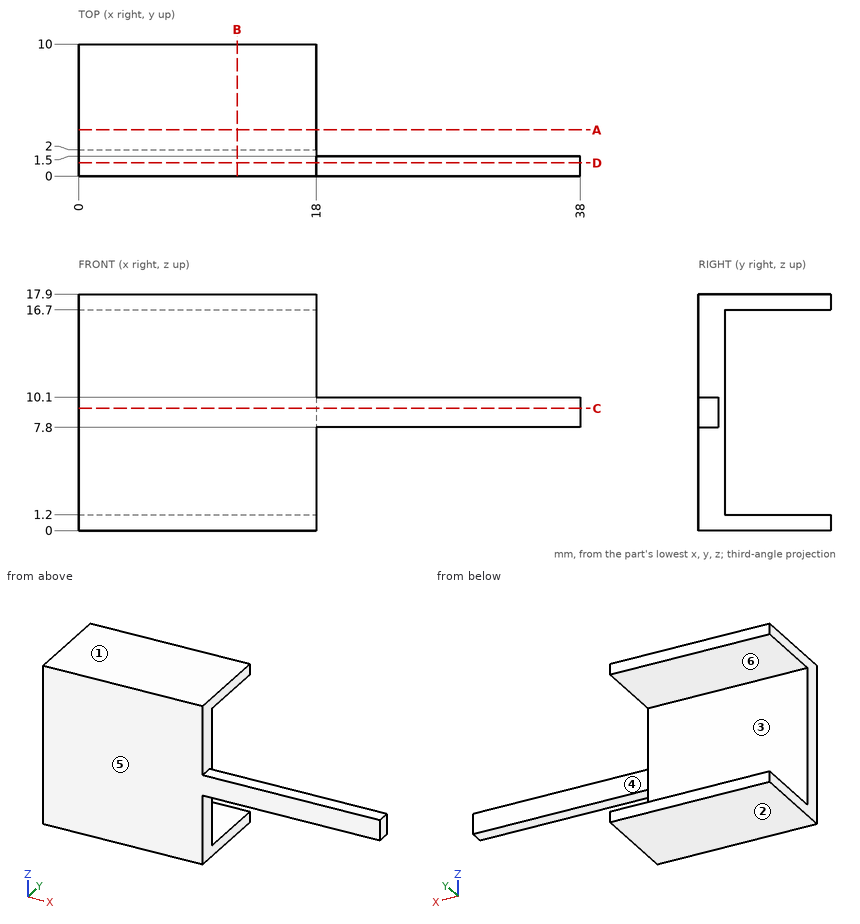
Design review of the part shown in the three views and the two pictorial views. Dimensions are in mm from the part's minimum x, y and z. A direction names the side the tool comes from. Give positions to 0.01 mm unless a question says otherwise; leave off trailing zeros. Loops run counter-clockwise (first coordinate to the right, second up) from the corner with the lowest first, then second, coordinate; pieces in that order, holes last. Notation, with made-up numbers: (-15.5, 70) -> (28.5, 70) arc R6 cw to (28.5, 76) -> close; hole circle Ø1 at (-18, 41). An arc over 180 degrees is marked (long way). Answer as a JSON object with one key per item and string values. Group by question number.
Q1. Draft analysis for pull direction Z (two halves, no side actions). For the marked faces 1, 2 and 3, state which applies: pulls with the +Z half, pulls with the -Z half, needs draft (parallel to the pull), parting line crosses it, or undercut.
Q2. Tool access review of the marked faces 4, 5 and 6: name each direction out of +Z, -Z, +X, -X, +Y, -Y from which nothing blocks a thin tool from reaching the whole face with its end or side.
Q3. Wall thickness on line 1 along Z through (x, y) = (4, 8); line 2 along Y through (x, z) = (11, 16); line 3 along X through (y, z) = (4.75, 17): over which ranges is each line inside the solid? List them lowest first.
Q4. Insertion check: pin 1 (1.6 mm diameter, centred on x = 25.5, y = 0.5, fed in from +Z); pin 2 (1.2 mm diameter, centred on x = 26, z = 9.5, fed in from +Y); pin 3 (1 mm diameter, centred on y = 1.5, z = 10.5, fed in from -X). Each pin has a flat end and moves straight along its axis. Give the tip position at first contact, or say it passes through.
Q5. Take a section at A-A (y = 3.5). Write out the cut boundary in (x, z).
Q6. Take a section at D-D (y = 1). Write out the cut boundary in (x, z), plus the area to 3 significant figures.
Q7. Take a section at B-B (x = 12). Write out the cut boundary in (y, z), plus the area to 3 significant figures.
Q8. Take a section at C-C (z = 9.25). Write out the cut boundary in (x, y), plus the area to 3 significant figures.
Answer below:
{
 "1": {"face 1": "pulls with the +Z half", "face 2": "pulls with the -Z half", "face 3": "undercut"},
 "2": {"face 4": "+Z, -Z, +X, +Y", "face 5": "+Z, -Z, +X, -X, -Y", "face 6": "+X, -X, +Y"},
 "3": {"line 1": "z = 0 to 1.2, 16.7 to 17.9", "line 2": "y = 0 to 2", "line 3": "x = 0 to 18"},
 "4": {"pin 1": "stops at z = 10.1", "pin 2": "stops at y = 1.5", "pin 3": "stops at x = 0"},
 "5": {"outline": "(0, 0) -> (18, 0) -> (18, 1.2) -> (0, 1.2) -> close; (0, 16.7) -> (18, 16.7) -> (18, 17.9) -> (0, 17.9) -> close"},
 "6": {"outline": "(0, 0) -> (18, 0) -> (18, 7.8) -> (38, 7.8) -> (38, 10.1) -> (18, 10.1) -> (18, 17.9) -> (0, 17.9) -> close", "area": "368 mm2"},
 "7": {"outline": "(0, 0) -> (10, 0) -> (10, 1.2) -> (2, 1.2) -> (2, 16.7) -> (10, 16.7) -> (10, 17.9) -> (0, 17.9) -> close", "area": "55.0 mm2"},
 "8": {"outline": "(0, 0) -> (38, 0) -> (38, 1.5) -> (18, 1.5) -> (18, 2) -> (0, 2) -> close", "area": "66.0 mm2"}
}
